Build history of the part. All positions in model axes, mm. Round coordinates to 2 decimals unless told otherwise and drop trailing zeros. Loops run counter-clockwise (first coordinate to the right, second up) from the corner with the lowest first, then second, coordinate; pieces in that order, holes last. Notation, with made-up numbers: (9.25, -9.75) -> (40.25, -9.75) arc R14 ccw to (40.25, 17.25) -> close; hole circle Ø8 at (4.5, -28.5). An arc over 180 degrees is marked (long way). Put each result on its own line as item: value. Start each with the question number.
Item 1: Drill centre lines: probe 1 along X at (y, z) = (2, 0); probe 2 along Y at (x, z) = (0.1, -0.35). Where is each one in solid material? Low to high. Write a range as [from, to].
Item 2: Cut at B-B, the plane x = 0. List the corners of the cut face in (y, z).
Item 3: Flat gauge pins, fed straight in: pin 1 Ø2 at (x, z) = (0.5, -0.5) entering from +Y; pin 2 Ø3 at (x, z) = (0, 0) entering from -Y. Where does each tip first touch, or does it go through?
Item 4: Cut at A-A, the plane z = 0. List the corners of the cut face in (x, y).
Item 5: Cut at C-C, the plane y = 69. List the corners of the cut face in (x, z).
```python
from build123d import *

# Parameters (mm, degrees)
SKETCH_1_R      = 3
SKETCH_1_R_2    = 2
EXTRUDE_1_DEPTH = 200
EXTRUDE_START   = -10
SKETCH_2_R      = 2
EXTRUDE_2_DEPTH = 3
SKETCH_3_R      = 2
EXTRUDE_3_DEPTH = 3


with BuildPart() as part:
    # 스케치1 → 보스-돌출1 (new body)
    with BuildSketch(Plane(origin=(0, 0, 0), x_dir=(1, 0, 0), z_dir=(0, 1, 0))):
        Circle(SKETCH_1_R)
        Circle(SKETCH_1_R_2, mode=Mode.SUBTRACT)
    extrude(amount=EXTRUDE_1_DEPTH)

    # 스케치2 → 보스-돌출2 (add)
    with BuildSketch(Plane.XZ.offset(EXTRUDE_START)):
        Circle(SKETCH_2_R)
    extrude(amount=-EXTRUDE_2_DEPTH)

    # 스케치3 → 보스-돌출3 (add)
    with BuildSketch(Plane(origin=(0, 200, 0), x_dir=(1, 0, 0), z_dir=(0, 1, 0)).offset(EXTRUDE_START)):
        Circle(SKETCH_3_R)
    extrude(amount=-EXTRUDE_3_DEPTH)


solid = part.part
```
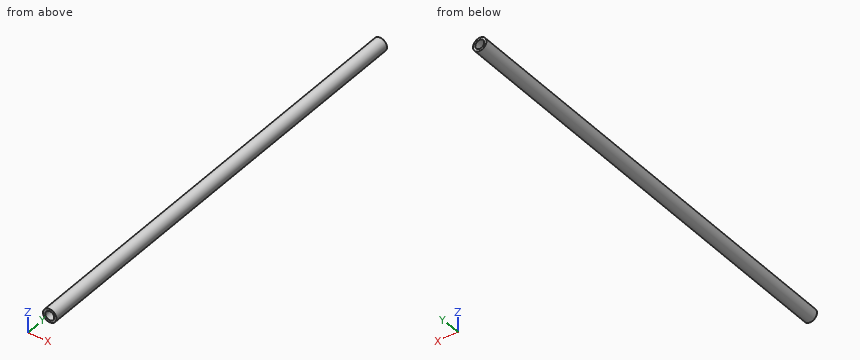
Reply:
1. probe 1: x = [-3, -2], [2, 3]
1. probe 2: y = [10, 13], [187, 190]
2. outline: (0, -3) -> (200, -3) -> (200, -2) -> (190, -2) -> (190, 2) -> (200, 2) -> (200, 3) -> (0, 3) -> (0, 2) -> (10, 2) -> (10, -2) -> (0, -2) -> close; hole (13, -2) -> (187, -2) -> (187, 2) -> (13, 2) -> close
3. pin 1: stops at y = 190
3. pin 2: stops at y = 10
4. outline: (-3, 0) -> (-2, 0) -> (-2, 10) -> (2, 10) -> (2, 0) -> (3, 0) -> (3, 200) -> (2, 200) -> (2, 190) -> (-2, 190) -> (-2, 200) -> (-3, 200) -> close; hole (-2, 13) -> (2, 13) -> (2, 187) -> (-2, 187) -> close
5. outline: circle Ø6 at (0, 0); hole circle Ø4 at (0, 0)
